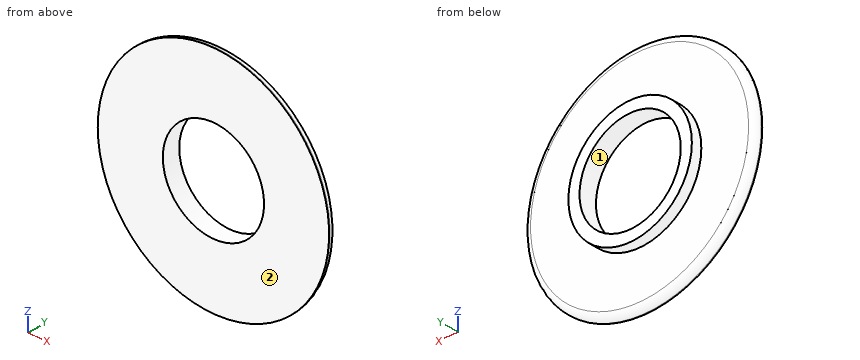
Autodesk Inventor part; units mm, degrees
ref_plane "YZ Plane" through (0, 0, 0) normal (1, 0, 0) x (0, 1, 0)
ref_plane "XZ Plane" through (0, 0, 0) normal (0, 1, 0) x (-1, 0, 0)
ref_plane "XY Plane" through (0, 0, 0) normal (0, 0, 1) x (1, 0, 0)
sketch "Sketch1" plane through (0, 0, 0) normal (0, 1, 0) x (-1, 0, 0)
  circle A0 centre (0, 0) radius 22.75
  circle A1 centre (0, 0) radius 52
  circle A2 centre (0, 0) radius 27.75
  dimension "d0" = 45.5
  dimension "d1" = 104
  dimension "d2" = 55.5
extrude "Extrusion1" add sketch "Sketch1" along normal blind 4.75 contours A2
extrude "Extrusion2" add sketch "Sketch1" against normal blind 3.5 contours A1 | A2
fillet "Fillet1" radius 3 1 edges at (52, 0, 0)
properties part number "motor_chain_guide_center"
Here's how the part is built. I have some questions about the finished solid (model axes, mm). Face numbers are marked on the shaded views. Coordinates: 2 decimals unless noted, no trailing zeros. Write each loop counter-clockwise with the first axis right and the second up, starting at its lowest first coordinate (ties: lowest second). Pieces come first, ordered by that corner, then holes. Notation, with made-up numbers: (17.25, 23) -> (23.25, 23) arc R13 cw to (23.25, 46) -> close; hole circle Ø8 at (-0.5, -4). An arc over 180 degrees is marked (long way). Use a Markdown table: item, result. Add a question column.
(1) If we section it at A-A, the plane z = 0: Write out the boundary of the cut face in (x, y), and give its area (3 significant figures).
(2) We'd pull the mould along Z, two halves only. Please class the marked faces 1 and 2: +Z half, -Z half, draft (parallel to the pull), parting line (faces both ways), or undercut.
(3) If we section it at B-B, the plane x = 0: Write out the boundary of the cut face in (y, z), and give its area (3 significant figures).
(4) If we section it at C-C, the plane y = 3.25: Write out the boundary of the cut face in (x, z), and give its area (3 significant figures).
(5) I'm going to push flat-ended pins straight in: P1, Ø6, axis at x = 32, z = 32, coming from the +Y side; P2, Ø1, axis at y = -1.5, z = -11, coming from the -X side; P3, Ø12, axis at x = -13.5, z = 0.5, coming from the -Y side; P4, Ø3, axis at y = 0.5, z = 31, coming from the +X side. Where does each tip first touch, or does it pass through?
(6) Please list where these lines run through material, in increasing order: line 1 (Z direction, x = 0, y = 2.25); line 2 (Y direction, x = -37, z = 28); line 3 (Z direction, x = -17, y = 0.25).
Outcome:
| question | item | result |
|---|---|---|
| 1 | outline | (-52, -3.5) -> (-22.75, -3.5) -> (-22.75, 4.75) -> (-27.75, 4.75) -> (-27.75, 0) -> (-49, 0) arc R3 ccw to (-52, -3) -> close; (22.75, -3.5) -> (52, -3.5) -> (52, -3) arc R3 ccw to (49, 0) -> (27.75, 0) -> (27.75, 4.75) -> (22.75, 4.75) -> close |
| 1 | area | 248 mm^2 |
| 2 | face 1 | undercut |
| 2 | face 2 | draft |
| 3 | outline | (-3.5, -52) -> (-3, -52) arc R3 ccw to (0, -49) -> (0, -27.75) -> (4.75, -27.75) -> (4.75, -22.75) -> (-3.5, -22.75) -> close; (-3.5, 22.75) -> (4.75, 22.75) -> (4.75, 27.75) -> (0, 27.75) -> (0, 49) arc R3 ccw to (-3, 52) -> (-3.5, 52) -> close |
| 3 | area | 248 mm^2 |
| 4 | outline | circle Ø55.5 at (0, 0); hole circle Ø45.5 at (0, 0) |
| 4 | area | 793 mm^2 |
| 5 | P1 | stops at y = 0 |
| 5 | P2 | stops at x = -50.68 |
| 5 | P3 | passes through |
| 5 | P4 | stops at x = 41.11 |
| 6 | line 1 | z = -27.75 to -22.75, 22.75 to 27.75 |
| 6 | line 2 | y = -3.5 to 0 |
| 6 | line 3 | z = -21.93 to -15.12, 15.12 to 21.93 |
